Check sheet for the modelled part. Datum: model origin and axes. Units: mm. A direction names the side the tool comes from. Give positions to 0.01 mm unless a question says otherwise; leave off trailing zeros. Write each loop counter-clockwise with the first axis right and the second up, starting at its lowest first coordinate (ties: lowest second). Pieces come first, ordered by that corner, then holes. Notation, with made-up numbers: (55, 62.5) -> (86, 62.5) arc R14 cw to (86, 70.5) -> close; hole circle Ø11 at (-8, 59.25). An arc over 180 degrees is marked (long way). Answer as a JSON object with one key per item and string values.
from build123d import *

# Parameters (mm, degrees)
F1_W     = 25.5
F1_H     = 12.5
F2_DEPTH = 26
F3_DEPTH = 24
F4_R     = 5
F5_R     = 1
F7_DEPTH = 1


with BuildPart() as f2:
    # F1 (on Top) → F2 (new body)
    with BuildSketch(Plane.XY):
        with Locations((0, -1.381356)):
            Rectangle(F1_W, F1_H)
    extrude(amount=F2_DEPTH)

    # F0 (on Top) → F3 (cut)
    with BuildSketch(Plane.XY):
        with BuildLine():
            Line((-5.25, -5.478824), (5.25, -5.478824))
            ThreePointArc((5.25, -5.478824), (8.078427, -4.307251), (9.25, -1.478824))
            Line((9.25, -1.478824), (9.25, -1.178824))
            ThreePointArc((9.25, -1.178824), (8.078427, 1.649603), (5.25, 2.821176))
            Line((5.25, 2.821176), (-5.25, 2.821176))
            ThreePointArc((-5.25, 2.821176), (-8.078427, 1.649603), (-9.25, -1.178824))
            Line((-9.25, -1.178824), (-9.25, -1.478824))
            ThreePointArc((-9.25, -1.478824), (-8.078427, -4.307251), (-5.25, -5.478824))
        make_face()
    extrude(amount=F3_DEPTH, mode=Mode.SUBTRACT)

    # F4
    f4_edges = [f2.edges().sort_by_distance(p)[0] for p in [
        (12.75, -7.631356, 13),
        (12.75, 4.868644, 13),
        (-12.75, -7.631356, 13),
        (-12.75, 4.868644, 13),
    ]]
    fillet(f4_edges, radius=F4_R)

    # F5
    f5_edges = [f2.edges().sort_by_distance(p)[0] for p in [
        (0, 4.868644, 0),
        (0, 4.868644, 26),
    ]]
    fillet(f5_edges, radius=F5_R)

    # F6 (on face) → F7 (join)
    with BuildSketch(Plane.XY):
        Polygon((-2.237371, -4.617726), (-3.124978, -5.505333), (3.585098, -5.505333), (2.697491, -4.617726), align=None)
    extrude(amount=F7_DEPTH)


solid = f2.part
1. Sectioned sample at D-D, the plane x = 7. Enter the section's corners in (y, z).
Determined:
{"outline": "(-7.63, 1) arc R1 ccw to (-6.63, 0) -> (-5.08, 0) -> (-5.08, 24) -> (2.42, 24) -> (2.42, 0) -> (3.87, 0) arc R1 ccw to (4.87, 1) -> (4.87, 25) arc R1 ccw to (3.87, 26) -> (-6.63, 26) arc R1 ccw to (-7.63, 25) -> close"}
2. Go/stop test with a flat-tipped pin: P1, Ø4, axis at x = 1, y = 0.5, coming from the -Z side. Record where the tip stops, or that it passes through.
Determined:
{"P1": "z = 24"}
3. Mould release check, pull along X, two halves, no side actions. Record for faces 1 (the face through (-12.449, -1.364, 0.285)), 2 (the face through (0, -5, 1)), 3 (the face through (0.108, 4.568, 0.285)): released by +X, released by -X, zero draft, split by the parting line, or undercut.
Determined:
{"face 1": "released by -X", "face 2": "undercut", "face 3": "zero draft"}
4. Access from +Z, -Z, +X, -X, +Y, -Y to the whole of each face (thin tool, end or side, straight path). Record for faces 4 (the face through (0, -5.479, 12)), 5 (the face through (11.246, -6.206, 13.168)), 6 (the face through (-2.66, -5.04, 0.49)).
Determined:
{"face 4": "none", "face 5": "+Z, -Z, +X, -Y", "face 6": "-Z"}
5. Sectioned sample at B-B, the plane x = 2.25. Enter the section's corners in (y, z).
Determined:
{"outline": "(-7.63, 1) arc R1 ccw to (-6.63, 0) -> (-4.62, 0) -> (-4.62, 1) -> (-5.48, 1) -> (-5.48, 24) -> (2.82, 24) -> (2.82, 0) -> (3.87, 0) arc R1 ccw to (4.87, 1) -> (4.87, 25) arc R1 ccw to (3.87, 26) -> (-6.63, 26) arc R1 ccw to (-7.63, 25) -> close"}
6. Scan lines: L1, parallel to X at y = -1, z = 14.75; L2, parallel to Y at x = -3.25, z = 1.5; L3, parallel to Z at x = -4.75, y = 2.5. Record each from-to range of solid material in increasing order. Write a range as [from, to].
Determined:
{"L1": "[-12.75, -9.25], [9.25, 12.75]", "L2": "[-7.63, -5.48], [2.82, 4.87]", "L3": "[24, 26]"}
7. Sectioned sample at A-A, the plane z = 19.75. Enter the section's corners in (x, y).
Determined:
{"outline": "(-12.75, -2.63) arc R5 ccw to (-7.75, -7.63) -> (7.75, -7.63) arc R5 ccw to (12.75, -2.63) -> (12.75, -0.13) arc R5 ccw to (7.75, 4.87) -> (-7.75, 4.87) arc R5 ccw to (-12.75, -0.13) -> close; hole (-9.25, -1.48) arc R4 ccw to (-5.25, -5.48) -> (5.25, -5.48) arc R4 ccw to (9.25, -1.48) -> (9.25, -1.18) arc R4 ccw to (5.25, 2.82) -> (-5.25, 2.82) arc R4 ccw to (-9.25, -1.18) -> close"}
8. Sectioned sample at C-C, the plane y = -0.5. Enter the section's corners in (x, z).
Determined:
{"outline": "(-12.75, 1) arc R1 ccw to (-11.75, 0) -> (-9.19, 0) -> (-9.19, 24) -> (9.19, 24) -> (9.19, 0) -> (11.75, 0) arc R1 ccw to (12.75, 1) -> (12.75, 25) arc R1 ccw to (11.75, 26) -> (-11.75, 26) arc R1 ccw to (-12.75, 25) -> close"}
